Input: dimensioned drawing with shaded views. Units: mm. Origin: part minimum x, y, z. A direction names the side the tool comes from. Round coordinates to 2 decimals unless told otherwise and drop trailing zeros. Order: outer loops, then holes, each group sorted by start corner. A loop starts at its lowest first (then second) coordinate and runs counter-clockwise, first axis right, second up. Notation, with made-up numbers: M 39.25,52.25 L 96.25,52.25 A8 cw 96.25,63.25 Z; hole C 88.5,-32.5 d4. An arc over 180 degrees is marked long. Put each result on its own line as item: value. Start each with the question number.
1) First-contact query: P1, Ø2, axis at x = 91.5, y = 38.5, coming from the -Z side; P2, Ø1.5, axis at x = 51.5, z = 25, coming from the +Y side; P3, Ø25, axis at x = 79.5, z = 82, coming from the +Y side. Flat tips, straight axial feed; report the tip coordinate or a pass-through.
2) Section B-B, the plane x = 113.5. Return loops of the section in (y, z), then the cut area to 4 significant figures.
3) Section D-D, the plane z = 97.5. Return loops of the section in (x, y).
4) Access query for the marked faces 1 and 2. Directions: +Z, -Z, +X, -X, +Y, -Y. A direction counts if a zero-diameter tool reaches every point of the face in a straight line with its end or side. Return the directions, or none.
5) Material intervals for probe 1 along Z at (x, y) = (94.5, 35.5); probe 2 along Z at (x, y) = (102, 19); probe 3 along X at (y, z) = (37.5, 36.5), sorted ascending. Write a range as [from, to].
6) Section A-A, the plane y = 8. Return loops of the section in (x, z).
7) Draft query along X for the marked faces 3, 4, 5 and 6. Return one class per face: pulls with the +X half, pulls with the -X half, needs draft (parallel to the pull), parting line crosses it, or undercut.
8) Section C-C, the plane z = 12. Return loops of the section in (x, y).
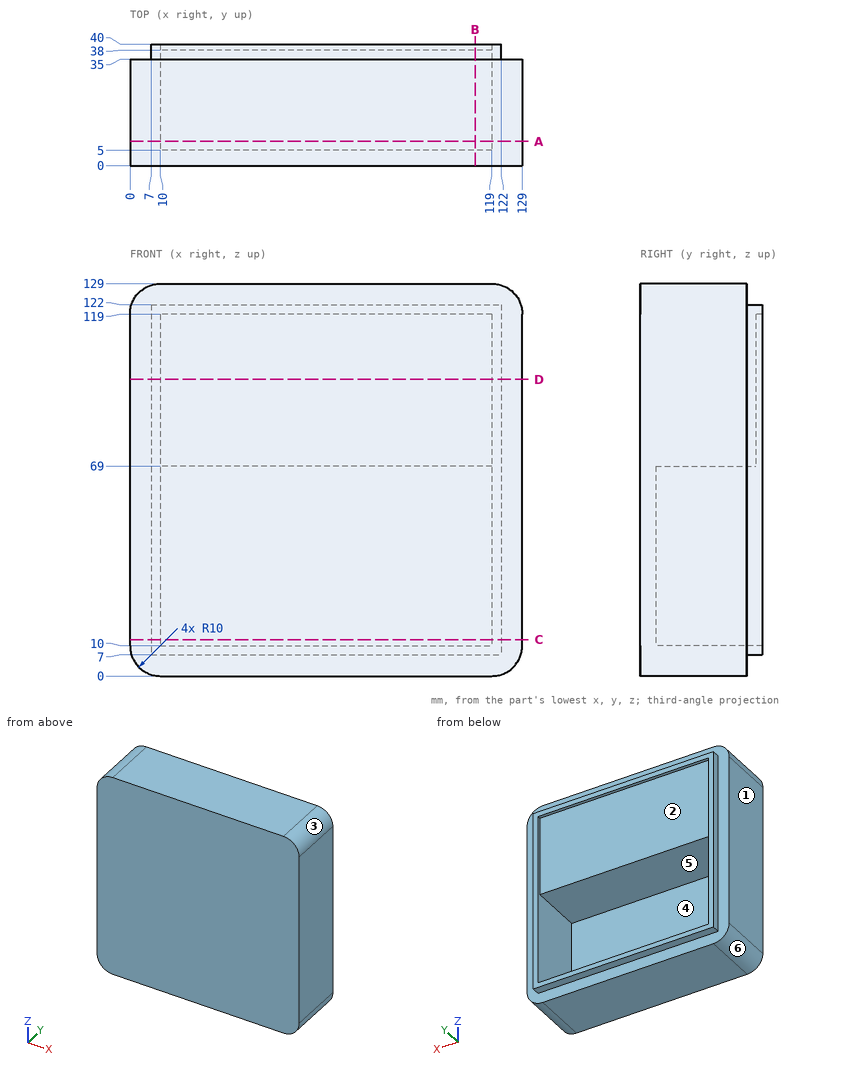
Result sheet:
1. P1: stops at z = 7
1. P2: stops at y = 5
1. P3: stops at y = 38
2. outline: M 0,0 L 35,0 L 35,7 L 40,7 L 40,10 L 5,10 L 5,69 L 38,69 L 38,119 L 40,119 L 40,122 L 35,122 L 35,129 L 0,129 Z
2. area: 2,925 mm2
3. outline: M 0,0 L 129,0 L 129,35 L 122,35 L 122,40 L 119,40 L 119,38 L 10,38 L 10,40 L 7,40 L 7,35 L 0,35 Z
4. face 1: +Z, -Z, -X, +Y, -Y
4. face 2: +Y
5. probe 1: z = [7, 10], [69, 122]
5. probe 2: z = [0, 10], [69, 129]
5. probe 3: x = [7, 10], [119, 122]
6. outline: M 0,10 A10 ccw 10,0 L 119,0 A10 ccw 129,10 L 129,119 A10 ccw 119,129 L 10,129 A10 ccw 0,119 Z; hole M 10,10 L 119,10 L 119,69 L 10,69 Z
7. face 3: pulls with the +X half
7. face 4: undercut
7. face 5: undercut
7. face 6: pulls with the -X half
8. outline: M 0,0 L 129,0 L 129,35 L 122,35 L 122,40 L 119,40 L 119,5 L 10,5 L 10,40 L 7,40 L 7,35 L 0,35 Z
